Autodesk Inventor part; units mm, degrees
ref_plane "YZ Plane" through (0, 0, 0) normal (1, 0, 0) x (0, 1, 0)
ref_plane "XZ Plane" through (0, 0, 0) normal (0, 1, 0) x (-1, 0, 0)
ref_plane "XY Plane" through (0, 0, 0) normal (0, 0, 1) x (1, 0, 0)
sketch "Sketch2" plane through (0, 0, 0) normal (0, 1, 0) x (-1, 0, 0)
  line L0 (0, 0) -> (105, 0)
  line L1 (105, 0) -> (105, -140)
  line L2 (105, -140) -> (0, -140)
  line L3 (0, -140) -> (0, 0)
  point P0 (75, -100)
  dimension "d4" = 105
  dimension "d5" = 140
extrude "Extrusion2" add sketch "Sketch2" along normal blind 3
sketch "Sketch3" plane through (0, 0, 0) normal (0, -1, 0) x (1, 0, 0)
  line L0 (-105, 0) -> (0, 0)
  line L1 (-105, -140) -> (-105, 0)
  line L2 (0, -17.5) -> (-3, -17.5)
  line L3 (-3, -17.5) -> (-3, -35)
  line L4 (-3, -35) -> (0, -35)
  line L5 (0, -35) -> (0, -52.5)
  line L6 (0, -52.5) -> (-3, -52.5)
  line L7 (-3, -52.5) -> (-3, -70)
  line L8 (-3, -70) -> (0, -70)
  line L9 (0, -70) -> (0, -87.5)
  line L10 (0, -87.5) -> (-3, -87.5)
  line L11 (-3, -87.5) -> (-3, -105)
  line L12 (-3, -105) -> (0, -105)
  line L13 (0, -105) -> (0, -122.5)
  line L14 (0, -122.5) -> (-3, -122.5)
  line L15 (-3, -122.5) -> (-3, -140)
  line L16 (0, -17.5) -> (0, 0)
  line L17 (-105, 0) -> (0, 0)
  line L18 (-105, -140) -> (-105, 0)
  line L19 (0, 0) -> (-105, 0)
  line L20 (-105, 0) -> (-105, -17.5)
  line L21 (-105, -17.5) -> (-102, -17.5)
  line L22 (-102, -17.5) -> (-102, -35)
  line L23 (-102, -35) -> (-105, -35)
  line L24 (-105, -35) -> (-105, -52.5)
  line L25 (-102, -52.5) -> (-105, -52.5)
  line L26 (-102, -52.5) -> (-102, -70)
  line L27 (-102, -70) -> (-105, -70)
  line L28 (-105, -70) -> (-105, -87.5)
  line L29 (-105, -87.5) -> (-102, -87.5)
  line L30 (-102, -87.5) -> (-102, -105)
  line L31 (-102, -105) -> (-105, -105)
  line L32 (-105, -105) -> (-105, -122.5)
  line L33 (-105, -122.5) -> (-102, -122.5)
  line L34 (-102, -122.5) -> (-102, -137)
  line L35 (0, -140) -> (-105, -140)
  line L36 (-105, -122.5) -> (-105, -105)
  line L37 (-102, -137) -> (-96.25, -137)
  line L38 (-96.25, -137) -> (-96.25, -140)
  line L39 (-96.25, -140) -> (-78.75, -140)
  line L40 (-52.5, -140) -> (-35, -140)
  line L41 (-17.5, -140) -> (-3, -140)
  line L42 (-3, -140) -> (-3, -137)
  line L43 (-61.25, -140) -> (-43.75, -140)
  line L44 (-43.75, -140) -> (-43.75, -137)
  line L45 (-43.75, -137) -> (-26.25, -137)
  line L46 (-26.25, -137) -> (-26.25, -140)
  line L47 (-26.25, -140) -> (-8.75, -140)
  line L48 (-8.75, -140) -> (-8.75, -137)
  line L49 (-8.75, -137) -> (-3, -137)
  line L50 (-96.25, -137) -> (-96.25, -140)
  line L51 (-96.25, -140) -> (-78.75, -140)
  line L52 (-78.75, -140) -> (-78.75, -137)
  line L53 (-78.75, -137) -> (-61.25, -137)
  line L54 (-61.25, -137) -> (-61.25, -140)
  line L55 (-61.25, -140) -> (-43.75, -140)
  line L56 (-26.25, -140) -> (-8.75, -140)
  point P0 (-17.5, -137)
  dimension "d51" = 3
  dimension "d52" = 17.5
  dimension "d53" = 17.5
  dimension "d54" = 17.5
  dimension "d55" = 17.5
  dimension "d56" = 17.5
  dimension "d58" = 3
  dimension "d65" = 17.5
  dimension "d66" = 17.5
  dimension "d67" = 17.5
  dimension "d69" = 5.75
  dimension "d70" = 5.75
  dimension "d71" = 17.5
extrude "Extrusion3" cut sketch "Sketch3" against normal blind 3 contours L0 L16 L2 L3 L4 L5 L6 L7 L8 L9 L10 L11 L12 L13 L14 L15 L49 L48 L35 L46 L45 L44 L54 L53 L52 L38 L37 L34 L33 L1 L31 L30 L29 L27 L26 L25 L23 L22 L21 keep common part
sketch "Sketch5" plane through (0, 3, 0) normal (0, 1, 0) x (1, 0, 0)
  circle A0 centre (-17.5, 17.5) radius 2.5
  line L0 (0, 0) -> (0, 17.5)
  line L1 (0, 0) -> (0, 17.5)
  line L2 (-105, 0) -> (0, 0)
  line L3 (0, 0) -> (-17.5, 0)
  circle A1 centre (-87.5, 17.5) radius 2.5
  circle A2 centre (-17.5, 122.5) radius 2.5
  circle A3 centre (-87.5, 122.5) radius 2.5
  dimension "d72" = 17.5
  dimension "d75" = 70
  dimension "d78" = 105
extrude "Extrusion4" cut sketch "Sketch5" against normal blind 2.5
properties part number "TableBottom" material "Wood (Cherry)"
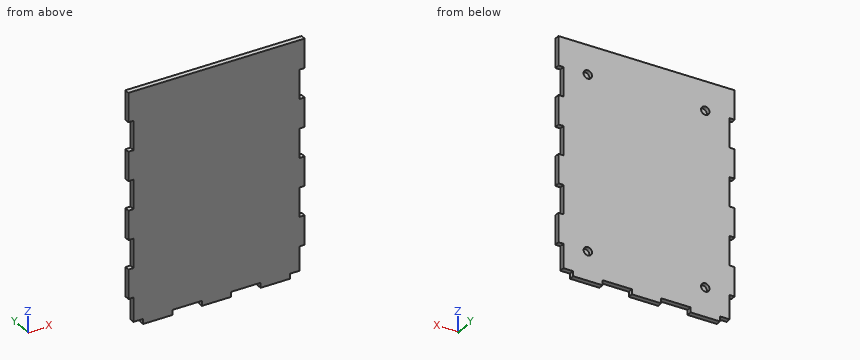
Geometry: final body of the model. Coordinates: model frame, mm. Round coordinates to 2 decimals unless told otherwise and drop trailing zeros. Loops run counter-clockwise (first coordinate to the right, second up) from the corner with the lowest first, then second, coordinate; pieces in that order, holes last. Notation, with made-up numbers: (-13.5, 14) - (10.5, 14) arc R18 ccw to (10.5, 46) - close; hole circle Ø7 at (-24, -14.5). An arc over 180 degrees is marked (long way). Write each question's results on one line, items separated by ' | '. Start each with the question number.
1) Line query: probe 1 along Z at (x, y) = (-17.5, 1.15); probe 2 along X at (y, z) = (2.25, -90.5); probe 3 along Z at (x, y) = (-3.5, 0.7). Output: solid intervals per line, ascending. Write a range as [from, to].
2) Cut plane B-B on y = 2.4. Count the separate pieces of the cut face and the enclosed holes in it, then the cut area to 3 significant figures.
3) Cut plane A-A on x = -87.5. Return loops of the section in (y, z), then the cut area to 3 significant figures.
4) First-contact query: P1, Ø8, axis at x = -83.5, z = -20, coming from the -Y side; P2, Ø0.9, axis at y = 1, z = -138, coming from the +X side; P3, Ø1.5, axis at y = 1.5, z = -98.5, coming from the -X side; P4, Ø1.5, axis at x = -16.5, z = -123.5, coming from the +Y side. Flat tips, straight axial feed; report the tip coordinate or a pass-through.
5) Cut plane C-C on z = -63. Return loops of the section in (x, y), then the cut area to 3 significant figures.
6) Cut plane D-D on x = -29. Return loops of the section in (y, z).
Verdict:
1) probe 1: z = [-140, -125], [-120, -20], [-15, 0] | probe 2: x = [-102, -3] | probe 3: z = [-137, 0]
2) separate pieces: 1 | enclosed holes: 4 | area: 14,100 mm2
3) outline: (0, -140) - (3, -140) - (3, -125) - (0.5, -125) - (0.5, -120) - (3, -120) - (3, -20) - (0.5, -20) - (0.5, -15) - (3, -15) - (3, 0) - (0, 0) - close | area: 395 mm2
4) P1: stops at y = 0 | P2: stops at x = -8.75 | P3: stops at x = -102 | P4: stops at y = 0.5
5) outline: (-102, 0) - (-3, 0) - (-3, 3) - (-102, 3) - close | area: 297 mm2
6) outline: (0, -137) - (3, -137) - (3, 0) - (0, 0) - close
